Drawing for the job (mm, zero at the part's lowest x, y, z). A direction names the side the tool comes from. Give positions to 0.01 mm unless a question says otherwise; leave off trailing zeros. Write each loop counter-clockwise with the first axis right and the second up, starting at its lowest first coordinate (ties: lowest second). Pieces come first, ordered by that corner, then holes. Notation, with made-up numbers: M -16,82.5 L 41,82.5 A4 ccw 41,88.5 Z; hole C 57,34 d2. An arc over 180 degrees is marked long. Use CSV: the item, a comma, the result in double quotes. Start each with the question number.
1. Drop flat-ended pins along their axis: pin 1 Ø0.8 at (y, z) = (1, 3) entering from -X; pin 2 Ø2 at (x, y) = (5, 11.5) entering from -Z; pin 3 Ø1.1 at (y, z) = (1.5, 3) entering from +X. Give the stop position or say it passes through.
2. Band-saw the part on C-C, the plane y = 11.5. List the corners of the cut face in (x, z), then the cut area to 3 significant figures.
3. Band-saw the part on D-D, the plane z = 4.4. List the corners of the cut face in (x, y).
4. 3-axis set-ups, long thin cutter, end or side, ignore diameter. For the marked faces 1, 2, 3 and 4: which of +Z, -Z, +X, -X, +Y, -Y reach the whole face in a straight line?
5. Band-saw the part on A-A, the plane z = 3. List the corners of the cut face in (x, y).
6. Drill centre lines: line 1 along Y through (x, z) = (5.35, 1.2); line 2 along Z through (x, y) = (2.65, 1) (3 decimals); line 3 along X through (y, z) = (2.75, 2.8). Where is each one in solid material? Low to high. Write a range as from..to.
7. Band-saw the part on B-B, the plane x = 2.6. List the corners of the cut face in (y, z) (1 decimal).
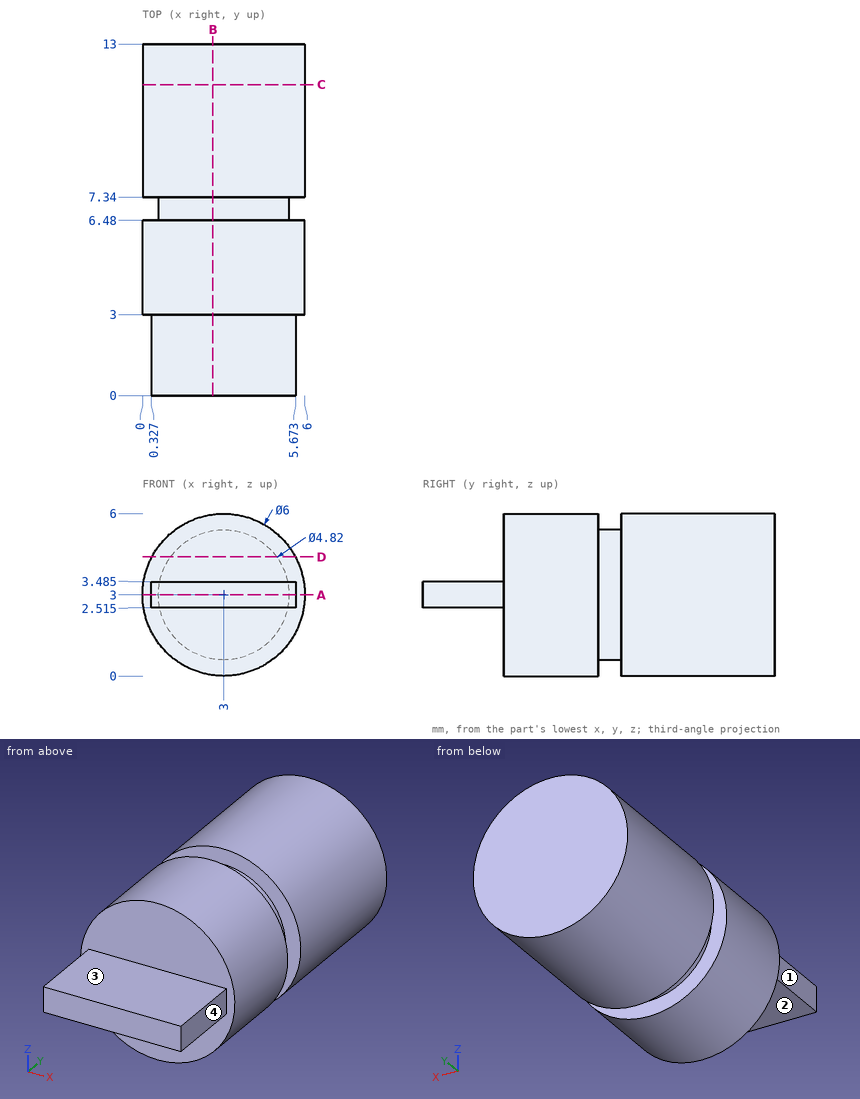
Output:
1,pin 1,"stops at x = 0.33"
1,pin 2,"stops at z = 0.17"
1,pin 3,"stops at x = 5.67"
2,outline,"C 3,3 d6"
2,area,"28.3 mm²"
3,outline,"M 0.35,3 L 5.65,3 L 5.65,6.48 L 4.96,6.48 L 4.96,7.34 L 5.65,7.34 L 5.65,13 L 0.35,13 L 0.35,7.34 L 1.04,7.34 L 1.04,6.48 L 0.35,6.48 Z"
4,face 1,"+Z, -Z, -X, -Y"
4,face 2,"-Z, +X, -X, -Y"
4,face 3,"+Z, +X, -X, -Y"
4,face 4,"+Z, -Z, +X, -Y"
5,outline,"M 0,3 L 0.33,3 L 0.33,0 L 5.67,0 L 5.67,3 L 6,3 L 6,6.48 L 5.41,6.48 L 5.41,7.34 L 6,7.34 L 6,13 L 0,13 L 0,7.34 L 0.59,7.34 L 0.59,6.48 L 0,6.48 Z"
6,line 1,"y = 3..6.48, 7.34..13"
6,line 2,"z = 2.515..3.485"
6,line 3,"x = 0.33..5.67"
7,outline,"M 0,2.5 L 3,2.5 L 3,0 L 6.5,0 L 6.5,0.6 L 7.3,0.6 L 7.3,0 L 13,0 L 13,6 L 7.3,6 L 7.3,5.4 L 6.5,5.4 L 6.5,6 L 3,6 L 3,3.5 L 0,3.5 Z"
